Input: part model. Units: mm. Frame: model coordinates. Face numbers are marked on the shaded views. A direction names the side the tool comes from. Coordinates: 2 decimals unless noted, no trailing zeros. Write each loop counter-clockwise with the first axis right and the second up, starting at its lowest first coordinate (ties: lowest second). Pieces come first, ordered by that corner, then holes. Notation, with made-up numbers: (34.25, -17.5) - (46.25, -17.5) arc R19 ccw to (46.25, 5.5) - close; hole circle Ø6 at (87.25, -25.75). An arc over 180 degrees is marked (long way). Put each result on its own line as item: value. Start each with the question number.
1. Cut plane A-A, the plane x = 31.5. Return loops of the section in (y, z).
2. Cut plane B-B, the plane z = -32. Return loops of the section in (x, y), and give its area (3 significant figures).
3. Line query: line 1 (Y direction, x = -19.5, z = 38); line 2 (Z direction, x = 9, y = 2.25); line 3 (Z direction, x = -4.5, y = 1.1). Output: solid intervals per line, ascending.
4. Access query for the marked faces 1, 2 and 3. Directions: +Z, -Z, +X, -X, +Y, -Y. A direction counts if a zero-diameter tool reaches every point of the face in a straight line with its end or side. Return the directions, or none.
5. Pin query (flat end, axial travel): pin 1 (3 mm diameter, centred on x = -5.5, y = 3, fed in from -Z); pin 2 (3.5 mm diameter, centred on x = -10.03, z = -44.29, fed in from +Y); pin 3 (1.9 mm diameter, centred on x = 10.67, z = -23.72, fed in from +Y); pin 4 (3 mm diameter, centred on x = 10, z = -12.5, fed in from -Y). Return the tip coordinate at first contact, or that it passes through.
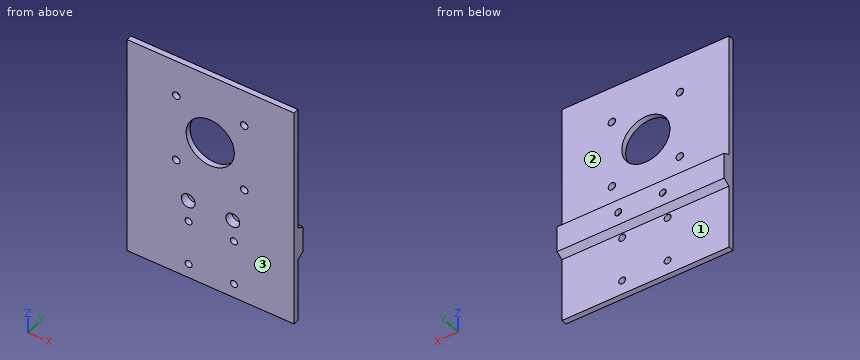
from build123d import *

# Parameters (mm, degrees)
SKETCH1_W           = 76.2
SKETCH1_H           = 101.6
BOSS_EXTRUDE1_DEPTH = 2.54
SKETCH2_R           = 1.5875
SKETCH2_R_2         = 1.70053
SKETCH2_R_3         = 10.99947
CUT_EXTRUDE1_DEPTH  = 2.54
BOSS_EXTRUDE2_DEPTH = 76.2
SKETCH4_R           = 3.175
CUT_EXTRUDE2_DEPTH  = 3.81
SKETCH5_R           = 1.5875
CUT_EXTRUDE3_DEPTH  = 3.032


with BuildPart() as part:
    # Sketch1 → Boss-Extrude1 (new body)
    with BuildSketch(Plane(origin=(0, 0, 0), x_dir=(1, 0, 0), z_dir=(0, 1, 0))):
        Rectangle(SKETCH1_W, SKETCH1_H)
    extrude(amount=BOSS_EXTRUDE1_DEPTH)

    # Sketch2 → Cut-Extrude1 (cut)
    with BuildSketch(Plane(origin=(0, 2.54, 0), x_dir=(1, 0, 0), z_dir=(0, 1, 0))):
        with Locations((-10.033800765, 44.29206639)):
            Circle(SKETCH2_R)
        with Locations((10.667199235, 44.29206639)):
            Circle(SKETCH2_R)
        with Locations((10.667199235, 23.71656639)):
            Circle(SKETCH2_R)
        with Locations((-10.033800765, 23.71656639)):
            Circle(SKETCH2_R)
        with Locations((-15.629995159, -3.207813583)):
            Circle(SKETCH2_R_2)
        with Locations((15.370704841, -3.207813583)):
            Circle(SKETCH2_R_2)
        with Locations((15.370704841, -34.208513583)):
            Circle(SKETCH2_R_2)
        with Locations((-15.629995159, -34.208513583)):
            Circle(SKETCH2_R_2)
        with Locations((-0.129645159, -18.708163583)):
            Circle(SKETCH2_R_3)
    extrude(amount=-CUT_EXTRUDE1_DEPTH, mode=Mode.SUBTRACT)

    # Sketch3 → Boss-Extrude2 (add)
    with BuildSketch(Plane(origin=(-38.1, 0, -50.8), x_dir=(0, 0, -1), z_dir=(1, 0, 0))):
        Polygon((-44.54593361, 2.54), (-29.30593361, 2.54), (-30.95693361, 5.842), (-42.89493361, 5.842), align=None)
    extrude(amount=BOSS_EXTRUDE2_DEPTH)

    # Sketch4 → Cut-Extrude2 (cut)
    with BuildSketch(Plane.XZ):
        with Locations((-10.16, -13.87406639)):
            Circle(SKETCH4_R)
        with Locations((10.16, -13.87406639)):
            Circle(SKETCH4_R)
    extrude(amount=-CUT_EXTRUDE2_DEPTH, mode=Mode.SUBTRACT)

    # Sketch5 → Cut-Extrude3 (cut, through all)
    with BuildSketch(Plane.XZ.offset(-3.81)):
        with Locations((-10.16, -13.87406639)):
            Circle(SKETCH5_R)
        with Locations((10.16, -13.87406639)):
            Circle(SKETCH5_R)
    extrude(amount=-CUT_EXTRUDE3_DEPTH, mode=Mode.SUBTRACT)


solid = part.part
Report:
1. outline: (0, -50.8) - (2.54, -50.8) - (2.54, -21.49) - (5.84, -19.84) - (5.84, -7.91) - (2.54, -6.25) - (2.54, 50.8) - (0, 50.8) - close
2. outline: (-38.1, 0) - (38.1, 0) - (38.1, 2.54) - (-38.1, 2.54) - close
2. area: 194 mm^2
3. line 1: y = 0 to 2.54
3. line 2: z = -50.8 to -16.83, -10.92 to 12.57, 24.84 to 50.8
3. line 3: z = -50.8 to 8.61, 28.8 to 50.8
4. face 1: -Z, +X, -X, +Y
4. face 2: +Z, +X, -X, +Y
4. face 3: +Z, -Z, +X, -X, -Y
5. pin 1: stops at z = -50.8
5. pin 2: stops at y = 2.54
5. pin 3: passes through
5. pin 4: stops at y = 3.81
